Model file for the job. Use its own axes, mm. Face numbers are marked on the shaded views. A direction names the side the tool comes from. Give positions to 0.01 mm unless a question says otherwise; leave off trailing zeros. Loops run counter-clockwise (first coordinate to the right, second up) from the corner with the lowest first, then second, coordinate; pieces in that order, holes last. Notation, with made-up numbers: (-24.5, -2.75) - (26.5, -2.75) arc R22 cw to (26.5, 17.25) - close; hole circle Ø8 at (-24, 21). An arc over 180 degrees is marked (long way). Answer as CSV lines item,"result". Start each with the question number.
Item 1: Pin check, flat tip, straight feed: pin 1 (1 mm diameter, centred on x = -5.5, z = -3.5, fed in from +Y). Stop position of the tip, or through.
Item 2: Pull direction Z, two halves, no side cores. Call the marked faces 3, 4 and 5: pulls with the +Z half, pulls with the -Z half, needs draft (parallel to the pull), parting line crosses it, or undercut.
Item 3: Saw through at A-A on y = 0.6. Give the cut face in (x, z).
Item 4: Drill centre lines: L1, parallel to X at y = 1.85, z = -27; L2, parallel to Z at x = -5, y = 2.7; L3, parallel to Z at x = -4, y = 0.8. Where is each one in solid material? Low to high. Write a range as from..to.
Item 5: Saw through at C-C on x = -5. Give the cut face in (y, z), plus the area to 3 significant figures.
Item 6: Tool access for the marked faces 1 and 2: list every direction of +Z, -Z, +X, -X, +Y, -Y with a clear straight run to the whole face (end or side of a thin tool).
Item 7: Saw through at B-B on z = -28. Give the cut face in (x, y).
Autodesk Inventor part; units mm, degrees
ref_plane "YZ Plane" through (0, 0, 0) normal (1, 0, 0) x (0, 1, 0)
ref_plane "XZ Plane" through (0, 0, 0) normal (0, 1, 0) x (-1, 0, 0)
ref_plane "XY Plane" through (0, 0, 0) normal (0, 0, 1) x (1, 0, 0)
sketch "Sketch1" plane through (0, 0, 0) normal (0, 1, 0) x (-1, 0, 0)
  line L0 (0, 0) -> (10, 0)
  line L1 (10, 0) -> (10, -32)
  line L2 (10, -32) -> (0, -32)
  line L3 (0, -32) -> (0, 0)
  line L4 (5, 0) -> (5, -4)
  line L5 (5, -32) -> (5, -29)
  line L6 (5, -4) -> (5, -29) construction
  line L7 (3.35, -4) -> (3.35, -29)
  line L8 (6.65, -29) -> (6.65, -4)
  arc A0 (6.65, -4) -> (3.35, -4) centre (5, -4) ccw
  arc A1 (3.35, -29) -> (6.65, -29) centre (5, -29) ccw
  point P0 (5, -16.5)
  dimension "d0" = 10
  dimension "d1" = 32
  dimension "d2" = 4
  dimension "d3" = 3
  dimension "d4" = 3.3
extrude "Extrusion1" add sketch "Sketch1" along normal blind 3 contours L0 L4 A0 L7 A1 L5 L2 L3 | L0 L1 L2 L5 A1 L8 A0 L4
properties part number "BeltMount2"
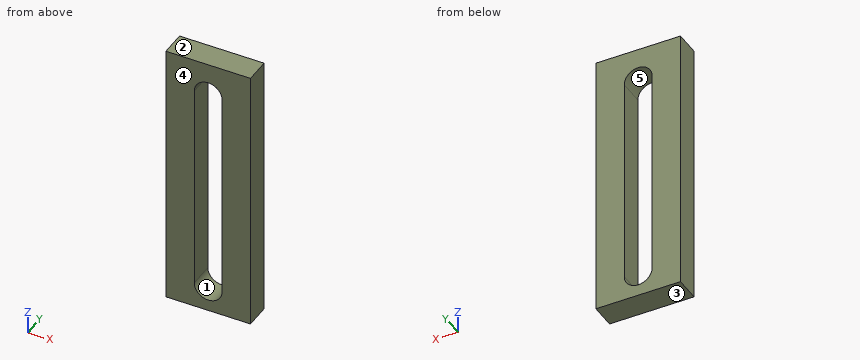
Responses:
1,pin 1,"through"
2,face 3,"pulls with the -Z half"
2,face 4,"needs draft"
2,face 5,"undercut"
3,outline,"(-10, -32) - (0, -32) - (0, 0) - (-10, 0) - close; hole (-6.65, -29) arc R1.65 ccw to (-3.35, -29) - (-3.35, -4) arc R1.65 ccw to (-6.65, -4) - close"
4,L1,"-10..-6.65, -3.35..0"
4,L2,"-32..-30.65, -2.35..0"
4,L3,"-32..-30.31, -2.69..0"
5,outline,"(0, -32) - (3, -32) - (3, -30.65) - (0, -30.65) - close; (0, -2.35) - (3, -2.35) - (3, 0) - (0, 0) - close"
5,area,"11.1 mm2"
6,face 1,"+Y, -Y"
6,face 2,"+Z, +X, -X, +Y, -Y"
7,outline,"(-10, 0) - (-6.65, 0) - (-6.65, 3) - (-10, 3) - close; (-3.35, 0) - (0, 0) - (0, 3) - (-3.35, 3) - close"
